Geometry check sheet. Reference: drawing and pictorial views, mm from the part's lowest x, y, z. A direction names the side the tool comes from. Give positions to 0.01 mm unless a question says otherwise; leave off trailing zeros. Loops run counter-clockwise (first coordinate to the right, second up) from the corner with the lowest first, then second, coordinate; pieces in that order, holes last. Notation, with made-up numbers: (50.5, 48) -> (103.5, 48) arc R15 cw to (103.5, 53) -> close; hole circle Ø10 at (-37, 10). An arc over 180 degrees is marked (long way). One line per item, written item: value. Start each with the question number.
(1) Gauge pin test, flat end, axial feed: pin 1 Ø3 at (x, y) = (15.47, 28.4) entering from +Z. Record the tip position at first contact, or that the pin passes through.
(2) Sectioned sample at C-C, the plane z = 8.25. Record the cut outline in (x, y) (1 decimal).
(3) Draft check along Z on the marked faces 3, 4 and 5. Enter one of: pulls with the +Z half, pulls with the -Z half, needs draft (parallel to the pull), parting line crosses it, or undercut.
(4) Tool access check on the marked faces 1 and 2. Record the directions out of +Z, -Z, +X, -X, +Y, -Y that give a thin tool (end or side, any length) a straight path to the whole face; none if there is none.
(5) Scan lines: line 1 along X through (y, z) = (43, 6.75) (1 decimal); line 2 along Z through (x, y) = (36, 38); line 3 along Z through (x, y) = (1, 38). Record each from-to range of solid material in increasing order. Write a range as from..to.
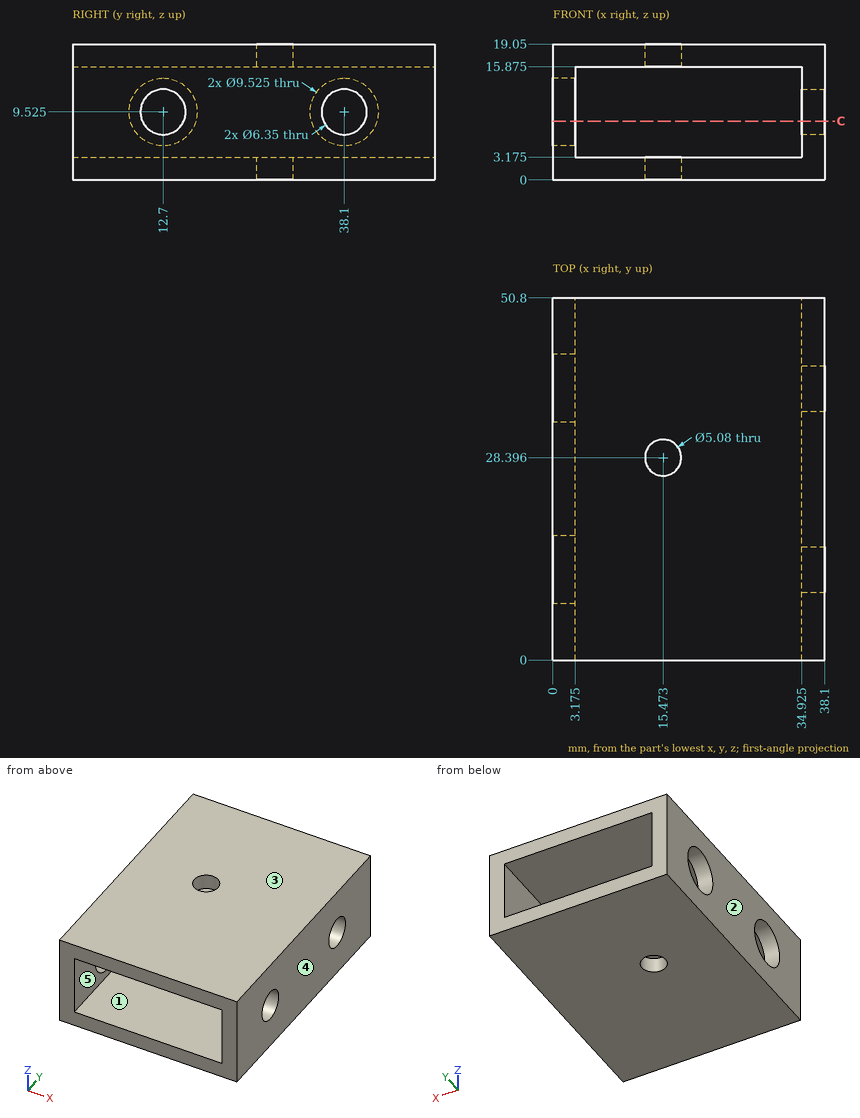
Calculated:
1. pin 1: passes through
2. outline: (0, 0) -> (3.2, 0) -> (3.2, 8.1) -> (0, 8.1) -> close; (0, 17.3) -> (3.2, 17.3) -> (3.2, 33.5) -> (0, 33.5) -> close; (0, 42.7) -> (3.2, 42.7) -> (3.2, 50.8) -> (0, 50.8) -> close; (34.9, 0) -> (38.1, 0) -> (38.1, 9.8) -> (34.9, 9.8) -> close; (34.9, 15.6) -> (38.1, 15.6) -> (38.1, 35.2) -> (34.9, 35.2) -> close; (34.9, 41) -> (38.1, 41) -> (38.1, 50.8) -> (34.9, 50.8) -> close
3. face 3: pulls with the +Z half
3. face 4: needs draft
3. face 5: undercut
4. face 1: +Y, -Y
4. face 2: +Z, -Z, -X, +Y, -Y
5. line 1: x = 0..3.2, 34.9..38.1
5. line 2: z = 0..6.35, 12.7..19.05
5. line 3: z = 0..4.76, 14.29..19.05
